Source: three-view drawing plus pictorial views. Frame: mm from the lowest corner of the part. A direction names the side the tool comes from. Give positions to 0.01 mm unless a question says otherwise; leave off trailing zeros. Write each loop counter-clockwise with the first axis right and the second up, starting at its lowest first coordinate (ties: lowest second). Pieces come first, ordered by that corner, then holes. Notation, with made-up numbers: (46, -24.75) -> (79, -24.75) arc R17 cw to (79, -19.75) -> close; hole circle Ø11 at (-36.75, -3). An arc over 180 degrees is marked (long way). Answer in a Markdown table with one row per item. Add a question column.
Item 1: Access query for the marked faces 1 and 2. Directions: +Z, -Z, +X, -X, +Y, -Y. A direction counts if a zero-diameter tool reaches every point of the face in a straight line with its end or side. Return the directions, or none.
Item 2: First-contact query: P1, Ø3, axis at y = 7.5, z = 31.5, coming from the -X side. Flat tip, straight axial feed; report the tip coordinate or a pass-through.
Item 3: Section query B-B on z = 10. Output: boundary loops of the cut face in (x, y).
Item 4: Section query A-A on y = 1. Output: boundary loops of the cut face in (x, z).
Item 5: Section query C-C on y = 10. Output: boundary loops of the cut face in (x, z).
Item 6: Material intervals for probe 1 along Y at (x, z) = (7.05, 10); probe 2 along Z at (x, y) = (7, 9.5); probe 3 along X at (y, z) = (10.5, 21), sorted ascending. Write a range as from..to.
Item 7: Section query D-D on z = 20. Output: boundary loops of the cut face in (x, y), plus the area to 3 significant figures.
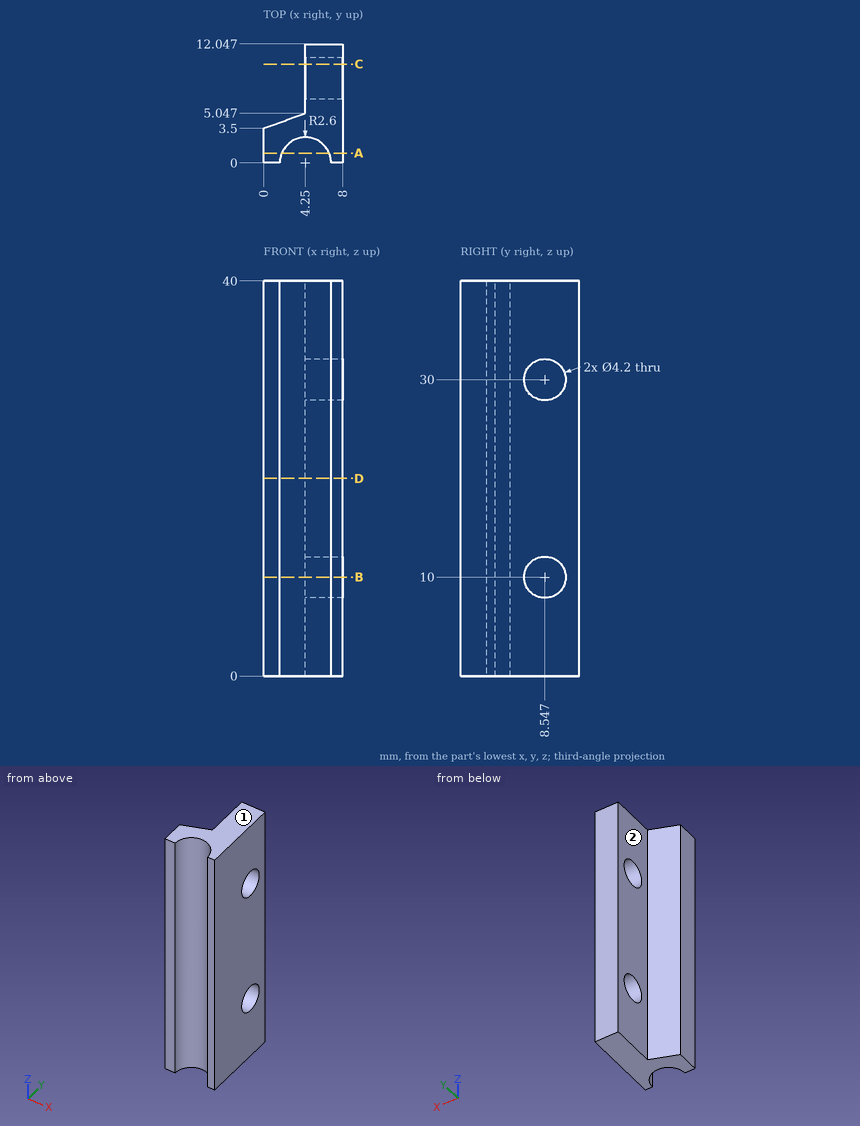
Findings below:
| question | item | result |
|---|---|---|
| 1 | face 1 | +Z, +X, -X, +Y, -Y |
| 1 | face 2 | +Z, -Z, -X, +Y |
| 2 | P1 | stops at x = 4.25 |
| 3 | outline | (0, 0) -> (1.65, 0) arc R2.6 cw to (6.85, 0) -> (8, 0) -> (8, 6.45) -> (4.25, 6.45) -> (4.25, 5.05) -> (0, 3.5) -> close; (4.25, 10.65) -> (8, 10.65) -> (8, 12.05) -> (4.25, 12.05) -> close |
| 4 | outline | (0, 0) -> (1.85, 0) -> (1.85, 40) -> (0, 40) -> close; (6.65, 0) -> (8, 0) -> (8, 40) -> (6.65, 40) -> close |
| 5 | outline | (4.25, 0) -> (8, 0) -> (8, 8.48) -> (4.25, 8.48) -> close; (4.25, 11.52) -> (8, 11.52) -> (8, 28.48) -> (4.25, 28.48) -> close; (4.25, 31.52) -> (8, 31.52) -> (8, 40) -> (4.25, 40) -> close |
| 6 | probe 1 | y = 0..6.45, 10.65..12.05 |
| 6 | probe 2 | z = 0..8.13, 11.87..28.13, 31.87..40 |
| 6 | probe 3 | x = 4.25..8 |
| 7 | outline | (0, 0) -> (1.65, 0) arc R2.6 cw to (6.85, 0) -> (8, 0) -> (8, 12.05) -> (4.25, 12.05) -> (4.25, 5.05) -> (0, 3.5) -> close |
| 7 | area | 52.7 mm^2 |
